from build123d import *

# Parameters (mm, degrees)
SKETCH1_W             = 40
SKETCH1_H             = 47.125
BOSS_EXTRUDE1_DEPTH   = 3.125
M4_CLEARANCE_HOLE1_D  = 4.3
M4X0_7_TAPPED_HOLE1_D = 3.3


with BuildPart() as part:
    # Sketch1 → Boss-Extrude1 (new body)
    with BuildSketch(Plane(origin=(0, 0, 0), x_dir=(1, 0, 0), z_dir=(0, 1, 0))):
        Rectangle(SKETCH1_W, SKETCH1_H)
    extrude(amount=BOSS_EXTRUDE1_DEPTH)

    # M4 Clearance Hole1 (through all)
    with Locations(Plane(origin=(0, 3.125, 0), x_dir=(1, 0, 0), z_dir=(0, 1, 0))):
        with Locations((16, -19.5625), (-16, -19.5625), (-16, 12.4375), (16, 12.4375)):
            Hole(M4_CLEARANCE_HOLE1_D / 2)

    # M4x0.7 Tapped Hole1 (through all)
    with Locations(Plane(origin=(0, 3.125, 0), x_dir=(1, 0, 0), z_dir=(0, 1, 0))):
        with Locations((0, -3.5625)):
            Hole(M4X0_7_TAPPED_HOLE1_D / 2)


solid = part.part
Can you work these out from the model? Positions are in its coordinate system, mm. Give positions to 0.01 mm unless a question says otherwise; leave off trailing zeros. Write each loop counter-clockwise with the first axis right and the second up, starting at its lowest first coordinate (ties: lowest second). Pieces come first, ordered by that corner, then holes. Notation, with made-up numbers: M 47.5,50 L 93.5,50 A12 ccw 93.5,64 Z; hole C 47.25,88 d11. An arc over 180 degrees is marked long. Answer in a Markdown table with one row per item. Add a question column.
Item 1: For pin 1 Ø3.5 at (x, z) = (16, 19.56) entering from +Y, with a flat end and sliding along its axis, tell me the tip position at first contact or that it passes through.
Item 2: Imagine slicing it at A-A, the plane x = -16. Write out the boundary of the cut face in (y, z) (1 decimal), plus the area to 3 significant figures.
Item 3: Imagine slicing it at B-B, the plane x = 0. Write out the boundary of the cut face in (y, z) (1 decimal), plus the area to 3 significant figures.
Item 4: Please list where these lines run through material, in increasing order: L1, parallel to Z at x = -16, y = 0.85; L2, parallel to X at y = 2.95, z = 19.5; L3, parallel to Z at x = 1.5, y = 0.8.
Item 5: Imagine slicing it at C-C, the plane y = 2. Write out the boundary of the cut face in (x, z), plus the area to 3 significant figures.
Item 6: We'd pull the mould along Z, two halves only. Please class faces 1 (the flat face through (0, 2, -23.562)), 2 (the cylindrical face through (-18.05, 1.54, -13.08)), 3 (the flat face through (20, 2, 0)), 4 (the flat face through (0, 2, 23.562)): released by +Z, released by -Z, zero draft, split by the parting line, or undercut.
Evaluation:
| question | item | result |
|---|---|---|
| 1 | pin 1 | passes through |
| 2 | outline | M 0,-23.6 L 3.1,-23.6 L 3.1,-14.6 L 0,-14.6 Z; M 0,-10.3 L 3.1,-10.3 L 3.1,17.4 L 0,17.4 Z; M 0,21.7 L 3.1,21.7 L 3.1,23.6 L 0,23.6 Z |
| 2 | area | 120 mm² |
| 3 | outline | M 0,-23.6 L 3.1,-23.6 L 3.1,1.9 L 0,1.9 Z; M 0,5.2 L 3.1,5.2 L 3.1,23.6 L 0,23.6 Z |
| 3 | area | 137 mm² |
| 4 | L1 | z = -23.56 to -14.59, -10.29 to 17.41, 21.71 to 23.56 |
| 4 | L2 | x = -20 to -18.15, -13.85 to 13.85, 18.15 to 20 |
| 4 | L3 | z = -23.56 to 2.88, 4.25 to 23.56 |
| 5 | outline | M -20,-23.56 L 20,-23.56 L 20,23.56 L -20,23.56 Z; hole C -16,-12.44 d4.3; hole C -16,19.56 d4.3; hole C 0,3.56 d3.3; hole C 16,-12.44 d4.3; hole C 16,19.56 d4.3 |
| 5 | area | 1,820 mm² |
| 6 | face 1 | released by -Z |
| 6 | face 2 | undercut |
| 6 | face 3 | zero draft |
| 6 | face 4 | released by +Z |
